Geometry check sheet. Reference: the model listing, model coordinates, mm. A direction names the side the tool comes from. Round coordinates to 2 decimals unless told otherwise and drop trailing zeros. Write each loop counter-clockwise with the first axis right and the second up, starting at its lowest first coordinate (ties: lowest second). Pieces come first, ordered by that corner, then holes. Notation, with made-up numbers: (2.25, -27.5) -> (57.25, -27.5) arc R19 cw to (57.25, -2.5) -> close; hole circle Ø5 at (15.5, -29.75). An arc over 180 degrees is marked (long way). Put each result on its own line as item: value. Start each with the question number.
from build123d import *

# Parameters (mm, degrees)
SKETCH1_R            = 50.8
BOSS_EXTRUDE1_DEPTH  = 101.6
SKETCH2_W            = 181.3814
SKETCH2_H            = 19.4056
SKETCH3_R            = 26.543
CUT_EXTRUDE1_DEPTH   = 216.526146906
SKETCH4_R            = 4.8895
CUT_EXTRUDE2_DEPTH   = 216.526146906
CIRPATTERN1_COUNT    = 6
FILLET1_R            = 3.175
BOSS_EXTRUDE2_DEPTH  = 50.8
CUT_EXTRUDE3_REACH   = 212.988
SKETCH6_R            = 3.302
LPATTERN1_COUNT      = 4
LPATTERN1_PITCH      = 25.4
LPATTERN1_COUNT_DIR2 = 2
LPATTERN1_PITCH_DIR2 = 25.4
CUT_EXTRUDE4_REACH   = 212.988
SKETCH7_R            = 3.302
LPATTERN2_COUNT      = 4
LPATTERN2_PITCH      = 25.4
LPATTERN2_COUNT_DIR2 = 2
LPATTERN2_PITCH_DIR2 = 25.4
FILLET2_R            = 1.5875
FILLET3_R            = 3.175


with BuildPart() as part:
    # Sketch1 → Boss-Extrude1 (new, symmetric)
    with BuildSketch(Plane.XY):
        Circle(SKETCH1_R)
    extrude(amount=BOSS_EXTRUDE1_DEPTH, both=True)

    # Sketch2 → Cut-Revolve1 (revolve, cut)
    with BuildSketch(Plane(origin=(0, 0, 0), x_dir=(0, 0, -1), z_dir=(1, 0, 0)), mode=Mode.PRIVATE) as cut_revolve1_sk:
        with Locations((1.1303, 41.0972)):
            Rectangle(SKETCH2_W, SKETCH2_H)
    revolve(cut_revolve1_sk.sketch.rotate(Axis((0, 0, -88.99), (0, 0, 1)), 90), axis=Axis((0, 0, -88.99), (0, 0, 1)), mode=Mode.SUBTRACT)

    # Sketch3 → Cut-Extrude1 (cut, through all)
    with BuildSketch(Plane.XY.offset(101.6)):
        Circle(SKETCH3_R)
    extrude(amount=-CUT_EXTRUDE1_DEPTH, mode=Mode.SUBTRACT)

    # Sketch4 → Cut-Extrude2 (cut, through all)
    with BuildSketch(Plane.XY.offset(101.6)):
        with Locations((0, 42.926)):
            Circle(SKETCH4_R)
    cut_extrude2 = extrude(amount=-CUT_EXTRUDE2_DEPTH, mode=Mode.SUBTRACT)

    # CirPattern1: Cut-Extrude2 ×6 about axis
    cirpattern1_axis = Axis((0, 0, 0), (0, 0, 1))
    for i in range(1, CIRPATTERN1_COUNT):
        add(cut_extrude2.rotate(cirpattern1_axis, i * 360 / CIRPATTERN1_COUNT), mode=Mode.SUBTRACT)

    # Fillet1
    fillet1_edges = [part.edges().sort_by_distance(p)[0] for p in [
        (31.3944, 0, 89.5604),
        (31.3944, 0, -91.821),
    ]]
    fillet(fillet1_edges, radius=FILLET1_R)

    # Sketch5 → Boss-Extrude2 (add, symmetric)
    with BuildSketch(Plane.XY):
        Polygon((28.9814, 3.175), (82.55, 3.175), (82.55, 25.4), (88.9, 25.4), (88.9, -25.4), (82.55, -25.4), (82.55, -3.175), (28.9814, -3.175), align=None)
        Polygon((-28.9814, -3.175), (-28.9814, 3.175), (-82.55, 3.175), (-82.55, 25.4), (-88.9, 25.4), (-88.9, -25.4), (-82.55, -25.4), (-82.55, -3.175), align=None)
    extrude(amount=BOSS_EXTRUDE2_DEPTH, both=True)

    # Sketch6 → Cut-Extrude3 (cut, up to next)
    with BuildSketch(Plane(origin=(88.9, 0, 0), x_dir=(0, 0, -1), z_dir=(1, 0, 0)), mode=Mode.PRIVATE) as cut_extrude3_sk1:
        with Locations((-38.1, -12.7)):
            Circle(SKETCH6_R)
    cut_extrude3_tool1 = extrude(cut_extrude3_sk1.sketch, amount=-CUT_EXTRUDE3_REACH, mode=Mode.PRIVATE) & part.part
    cut_extrude3 = cut_extrude3_tool1.solids().sort_by_distance((88.9, -12.7, 38.1))[0]
    add(cut_extrude3, mode=Mode.SUBTRACT)

    # LPattern1: Cut-Extrude3 4 × 2
    with Locations(*[(0, j * LPATTERN1_PITCH_DIR2, -i * LPATTERN1_PITCH) for i in range(LPATTERN1_COUNT) for j in range(LPATTERN1_COUNT_DIR2) if (i, j) != (0, 0)]):
        add(cut_extrude3, mode=Mode.SUBTRACT)

    # Sketch7 → Cut-Extrude4 (cut, up to next)
    with BuildSketch(Plane.ZY.offset(88.9), mode=Mode.PRIVATE) as cut_extrude4_sk1:
        with Locations(Location((38.1, -12.7, 0), (0, 0, 180))):
            Circle(SKETCH7_R)
    cut_extrude4_tool1 = extrude(cut_extrude4_sk1.sketch, amount=-CUT_EXTRUDE4_REACH, mode=Mode.PRIVATE) & part.part
    cut_extrude4 = cut_extrude4_tool1.solids().sort_by_distance((-88.9, -12.7, 38.1))[0]
    add(cut_extrude4, mode=Mode.SUBTRACT)

    # LPattern2: Cut-Extrude4 4 × 2
    with Locations(*[(0, j * LPATTERN2_PITCH_DIR2, -i * LPATTERN2_PITCH) for i in range(LPATTERN2_COUNT) for j in range(LPATTERN2_COUNT_DIR2) if (i, j) != (0, 0)]):
        add(cut_extrude4, mode=Mode.SUBTRACT)

    # Fillet2
    fillet2_edges = [part.edges().sort_by_distance(p)[0] for p in [
        (82.55, 3.175, 0),
        (82.55, -3.175, 0),
        (-82.55, -3.175, 0),
        (-82.55, 3.175, 0),
    ]]
    fillet(fillet2_edges, radius=FILLET2_R)

    # Fillet3
    fillet3_edges = [part.edges().sort_by_distance(p)[0] for p in [
        (31.3944, 0, -50.8),
        (31.233439234, 3.175, 0),
        (31.233439234, -3.175, 0),
        (31.3944, 0, 50.8),
        (-31.354133986, -1.58953872, -50.8),
        (-31.233439234, 3.175, 0),
        (-31.233439234, -3.175, 0),
        (-31.354133986, -1.58953872, 50.8),
    ]]
    fillet(fillet3_edges, radius=FILLET3_R)


solid = part.part
(1) Sectioned sample at C-C (z = -12.7). State how many separate pieces and enclosed holes the cut face has, and give its area (3 significant figures).
(2) Set-up check for faces 1 (the flat face through (82.55, 15, -1)), 2 (the cylindrical face through (85.77, 15.48, -39.88)), 3 (the cylindrical face through (-29.945, -9.43, -2.356)): record each of +Z, -Z, +X, -X, +Y, -Y from which the full face is reachable in a straight line by a thin tool's end or side.
(3) Mould release check, pull along X, two halves, no side actions. Record for faces 4 (the flat face through (-82.55, -15, 1)), 5 (the flat face through (-72, 0, 50.8)), 6 (the cylindrical face through (-11.012, -49.592, -96.642)): +X half, -X half, draft (parallel to the pull), parting line (faces both ways), or undercut.
(4) Sectioned sample at D-D (x = -48). Record the cut outline in (y, z) (1 decimal).
(5) Material ranges on L1, parallel to Z at x = -86.5, y = -12.7; L2, parallel to X at y = 19, z = 33; L3, parallel to Y at x = 0, z = -30, recorded low to high. Write a range as from..to.
(6) Go/stop test with flat-tipped pins: pin 1 Ø1.9 at (x, z) = (-84, -8) entering from -Y; pin 2 Ø6 at (y, z) = (-12.7, -12.7) entering from -X; pin 3 Ø12 at (x, z) = (11, -58.5) entering from -Y; pin 4 Ø6 at (x, y) = (-37.18, 21.46) entering from -Z. Record where each tip stops, or that it passes through.
Found:
1. separate pieces: 5
1. enclosed holes: 1
1. area: 2,020 mm2
2. face 1: +Z, -Z, +Y
2. face 2: +X
2. face 3: none
3. face 4: undercut
3. face 5: draft
3. face 6: parting line
4. outline: (-16.6, -101.6) -> (16.6, -101.6) -> (16.6, -91.8) -> (-16.6, -91.8) -> close; (-16.6, 89.6) -> (16.6, 89.6) -> (16.6, 101.6) -> (-16.6, 101.6) -> close; (-3.2, -50.8) -> (3.2, -50.8) -> (3.2, 50.8) -> (-3.2, 50.8) -> close
5. L1: -50.8..-41.4, -34.8..-16, -9.4..9.4, 16..34.8, 41.4..50.8
5. L2: -88.9..-82.55, -24.99..-18.53, 18.53..24.99, 82.55..88.9
5. L3: -31.39..-26.54, 26.54..31.39
6. pin 1: y = -25.4
6. pin 2: x = -29.86
6. pin 3: y = -30.99
6. pin 4: through
